Input: part model. Units: mm. Frame: model coordinates. Face numbers are marked on the shaded views. A direction names the side the tool comes from. Round coordinates to 2 decimals unless told otherwise and drop trailing zeros. Order: outer loops, then holes, each group sorted by start corner. A loop starts at its lowest first (then second) coordinate and runs counter-clockwise, first axis right, second up.
Item 1: Mould query, pull axis Y, two halves, no side actions, for the marked faces 1, 2 and 3. Classes: released by +Y, released by -Y, zero draft, split by the parting line, or undercut.
Item 2: Cut plane D-D on z = 12. Output: boundary loops of the cut face in (x, y).
Item 3: Cut plane C-C on x = 13.5. Output: boundary loops of the cut face in (y, z), then the cut area to 3 significant figures.
Item 4: Cut plane B-B on y = 11.75. Output: boundary loops of the cut face in (x, z).
Item 5: Reachability of the marked faces 4, 5, 6 and 7 from +Z, -Z, +X, -X, +Y, -Y: full face, straight path, thin tool, end or side. Return the list, or none.
Item 6: Cut plane A-A on y = 5.25. Give the number of separate pieces and of enclosed holes in the cut face, then the cut area to 3 significant figures.
Item 7: First-contact query: pin 1 (12.5 mm diameter, centred on x = 35, z = -25, fed in from +Y); pin 2 (3 mm diameter, centred on y = 18.5, z = 11.5, fed in from +X). Flat tips, straight axial feed; report the tip coordinate or a pass-through.
Item 8: Line query: L1, parallel to X at y = 9, z = 1.5; L2, parallel to X at y = 2.75, z = 9; L3, parallel to X at y = 11.5, z = 1. Output: solid intervals per line, ascending.
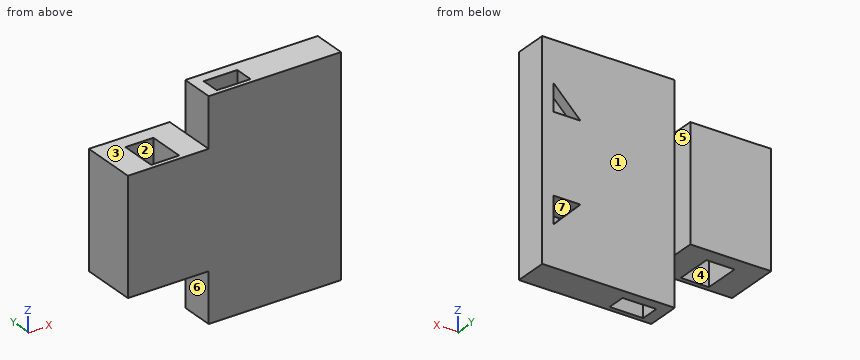
```python
from build123d import *

# Parameters (mm, degrees)
SKETCH1_W           = 90
SKETCH1_H           = 95
BOSS_EXTRUDE3_DEPTH = 15
SKETCH5_W           = 15
SKETCH5_H           = 8.4
CUT_EXTRUDE3_DEPTH  = 40
SKETCH7_W           = 95
SKETCH7_H           = 15
BOSS_EXTRUDE4_DEPTH = 5
CUT_EXTRUDE7_DEPTH  = 13
SKETCH12_W          = 15
SKETCH12_H          = 8.4
CUT_EXTRUDE8_DEPTH  = 20
CUT_EXTRUDE9_DEPTH  = 13
SKETCH14_W          = 15
SKETCH14_H          = 8.4
CUT_EXTRUDE11_DEPTH = 20
SKETCH15_W          = 36
SKETCH15_H          = 15
CUT_EXTRUDE12_DEPTH = 22
SKETCH16_W          = 36
SKETCH16_H          = 15
CUT_EXTRUDE13_DEPTH = 22
SKETCH17_W          = 36
SKETCH17_H          = 51
BOSS_EXTRUDE5_DEPTH = 10
SKETCH18_W          = 12.5
SKETCH18_H          = 16.5
CUT_EXTRUDE14_DEPTH = 100
SKETCH19_W          = 15
SKETCH19_H          = 8.4
CUT_EXTRUDE15_DEPTH = 100


with BuildPart() as part:
    # Sketch1 → Boss-Extrude3 (new body)
    with BuildSketch(Plane(origin=(0, 0, 0), x_dir=(1, 0, 0), z_dir=(0, 1, 0))):
        Rectangle(SKETCH1_W, SKETCH1_H)
    extrude(amount=BOSS_EXTRUDE3_DEPTH)

    # Sketch5 → Cut-Extrude3 (cut)
    with BuildSketch(Plane(origin=(45, 0, 0), x_dir=(0, 0, -1), z_dir=(1, 0, 0))):
        with Locations((0.9, 6.2)):
            Rectangle(SKETCH5_W, SKETCH5_H)
    extrude(amount=-CUT_EXTRUDE3_DEPTH, mode=Mode.SUBTRACT)

    # Sketch7 → Boss-Extrude4 (add)
    with BuildSketch(Plane(origin=(45, 0, 0), x_dir=(0, 0, -1), z_dir=(1, 0, 0))):
        with Locations((0, 7.5)):
            Rectangle(SKETCH7_W, SKETCH7_H)
    extrude(amount=BOSS_EXTRUDE4_DEPTH)

    # Sketch10 → Cut-Extrude7 (cut)
    with BuildSketch(Plane(origin=(0, 15, 0), x_dir=(1, 0, 0), z_dir=(0, 1, 0))):
        Polygon((33, -17.5), (45, -17.5), (45, -29.5), align=None)
    extrude(amount=-CUT_EXTRUDE7_DEPTH, mode=Mode.SUBTRACT)

    # Sketch12 → Cut-Extrude8 (cut)
    with BuildSketch(Plane(origin=(7.75, 0, -7.75), x_dir=(-0.707106781, 0, -0.707106781), z_dir=(0.707106781, 0, -0.707106781))):
        with Locations((-44.20889245, 6.2)):
            Rectangle(SKETCH12_W, SKETCH12_H)
    extrude(amount=-CUT_EXTRUDE8_DEPTH, mode=Mode.SUBTRACT)

    # Sketch13 → Cut-Extrude9 (cut)
    with BuildSketch(Plane(origin=(0, 15, 0), x_dir=(1, 0, 0), z_dir=(0, 1, 0))):
        Polygon((33, 17.5), (45, 17.5), (45, 29.5), align=None)
    extrude(amount=-CUT_EXTRUDE9_DEPTH, mode=Mode.SUBTRACT)

    # Sketch14 → Cut-Extrude11 (cut)
    with BuildSketch(Plane(origin=(7.75, 0, 7.75), x_dir=(0.707106781, 0, -0.707106781), z_dir=(0.707106781, 0, 0.707106781))):
        with Locations((44.20889245, 6.2)):
            Rectangle(SKETCH14_W, SKETCH14_H)
    extrude(amount=-CUT_EXTRUDE11_DEPTH, mode=Mode.SUBTRACT)

    # Sketch15 → Cut-Extrude12 (cut)
    with BuildSketch(Plane.XY.offset(47.5)):
        with Locations((-27, 7.5)):
            Rectangle(SKETCH15_W, SKETCH15_H)
    extrude(amount=-CUT_EXTRUDE12_DEPTH, mode=Mode.SUBTRACT)

    # Sketch16 → Cut-Extrude13 (cut)
    with BuildSketch(Plane(origin=(0, 0, -47.5), x_dir=(-1, 0, 0), z_dir=(0, 0, -1))):
        with Locations((27, 7.5)):
            Rectangle(SKETCH16_W, SKETCH16_H)
    extrude(amount=-CUT_EXTRUDE13_DEPTH, mode=Mode.SUBTRACT)

    # Sketch17 → Boss-Extrude5 (add)
    with BuildSketch(Plane(origin=(0, 15, 0), x_dir=(1, 0, 0), z_dir=(0, 1, 0))):
        with Locations((-27, 0)):
            Rectangle(SKETCH17_W, SKETCH17_H)
    extrude(amount=BOSS_EXTRUDE5_DEPTH)

    # Sketch18 → Cut-Extrude14 (cut)
    with BuildSketch(Plane(origin=(0, 0, -25.5), x_dir=(-1, 0, 0), z_dir=(0, 0, -1))):
        with Locations((27, 10.25)):
            Rectangle(SKETCH18_W, SKETCH18_H)
    extrude(amount=-CUT_EXTRUDE14_DEPTH, mode=Mode.SUBTRACT)

    # Sketch19 → Cut-Extrude15 (cut)
    with BuildSketch(Plane(origin=(0, 0, -47.5), x_dir=(-1, 0, 0), z_dir=(0, 0, -1))):
        with Locations((-3.5, 6.2)):
            Rectangle(SKETCH19_W, SKETCH19_H)
    extrude(amount=-CUT_EXTRUDE15_DEPTH, mode=Mode.SUBTRACT)


solid = part.part
```
From the geometry:
1. face 1: released by +Y
1. face 2: undercut
1. face 3: zero draft
2. outline: (-45, 0) - (50, 0) - (50, 15) - (-9, 15) - (-9, 25) - (-45, 25) - close; hole (-33.25, 2) - (-20.75, 2) - (-20.75, 18.5) - (-33.25, 18.5) - close; hole (-4, 2) - (11, 2) - (11, 10.4) - (-4, 10.4) - close
3. outline: (0, -47.5) - (15, -47.5) - (15, 47.5) - (0, 47.5) - close; hole (2, -8.4) - (10.4, -8.4) - (10.4, 6.6) - (2, 6.6) - close
3. area: 1,300 mm2
4. outline: (-45, -25.5) - (-33.25, -25.5) - (-33.25, 25.5) - (-45, 25.5) - close; (-20.75, -25.5) - (-9, -25.5) - (-9, -47.5) - (50, -47.5) - (50, 47.5) - (-9, 47.5) - (-9, 25.5) - (-20.75, 25.5) - close; hole (33, -17.5) - (45, -29.5) - (45, -17.5) - close; hole (33, 17.5) - (45, 17.5) - (45, 29.5) - close
5. face 4: +Z, -Z
5. face 5: +Z, -Z, +X, +Y
5. face 6: -Z, -X, +Y, -Y
5. face 7: +Y
6. separate pieces: 3
6. enclosed holes: 2
6. area: 4,120 mm2
7. pin 1: stops at y = 15
7. pin 2: stops at x = -9
8. L1: x = -45 to -33.25, -20.75 to -4, 45 to 50
8. L2: x = -45 to -33.25, -20.75 to -4, 11 to 50
8. L3: x = -45 to -33.25, -20.75 to 50
